Here's how the part is built. I have some questions about the finished solid (model axes, mm). Face numbers are marked on the shaded views. A direction names the side the tool comes from. Round coordinates to 2 decimals unless told otherwise and drop trailing zeros. Write each loop counter-clockwise with the first axis right and the second up, starting at its lowest first coordinate (ties: lowest second). Pieces come first, ordered by that corner, then holes. Notation, with made-up numbers: (27, 37) - (83, 37) arc R31 ccw to (83, 75) - close; hole circle Ø5 at (18, 17.25). An arc over 180 degrees is marked (long way). Write item = value, one per line. Start each with the question number.
Item 1: If we section it at D-D (x = 4): Please give me the cut outline in (y, z).
Item 2: If we section it at B-B (z = -88): Please give me the cut outline in (x, y), and give its area (3 significant figures).
Item 3: Which directions (+Z, -Z, +X, -X, +Y, -Y) give clear straight access to the entire face, cutting with the end or side of a thin tool? Please do the marked faces 1 and 2.
Item 4: If I drill on line 1 along X through (y, z) = (26, -39); line 2 along Y through (x, z) = (178, 8); line 3 along Z through (x, y) = (21, -136.5), over which ranges is the centre line in solid material (lowest first)? Write a range as [from, to].
Item 5: If we section it at A-A (x = -57.5): Please give me the cut outline in (y, z).
Item 6: For P1, Ø5, axis at x = -16, y = -50.5, coming from the -Z side; P2, Ø8, axis at y = -79.5, z = -106.5, coming from the -X side, each with a flat end and sliding along its axis, tell me the tip position at first contact or that it passes through.
Item 7: If we section it at C-C (y = -17.5): Please give me the cut outline in (x, z), and give its area (3 significant figures).
```python
from build123d import *

# Parameters (mm, degrees)
F0_W      = 406.4
F0_H      = 203.2
F1_DEPTH  = 101.6
F4_W      = 393.7
F4_H      = 190.5
F5_DEPTH  = 190.5
F6_R      = 38.1
F7_DEPTH  = 6.35
F10_DEPTH = 101.6


# Not quite as in the source:
# - the program builds the solid bodies; features that only make, move or delete a surface that nothing else refers to are left out


with BuildPart() as f1:
    # F0 (on Top) → F1 (new body, symmetric)
    with BuildSketch(Plane.XY):
        with Locations((-1.672681421, -62.5133958211)):
            Rectangle(F0_W, F0_H)
    extrude(amount=F1_DEPTH, both=True)

    # F4 (on offset) → F5 (cut)
    with BuildSketch(Plane.XZ.offset(157.7633958211)):
        with Locations((-1.672681421, 0)):
            Rectangle(F4_W, F4_H)
    extrude(amount=-F5_DEPTH, mode=Mode.SUBTRACT)

    # F6 (on face) → F7 (cut, through all)
    with BuildSketch(Plane(origin=(0, 0, -101.6), x_dir=(1, 0, 0), z_dir=(0, 0, -1))):
        with Locations((13.9572741464, 5.3633958211)):
            Circle(F6_R)
    extrude(amount=-F7_DEPTH, mode=Mode.SUBTRACT)

    # F9 (on offset) → F10 (join)
    with BuildSketch(Plane(origin=(0, 0, -95.25), x_dir=(1, 0, 0), z_dir=(0, 0, -1))):
        with BuildLine():
            ThreePointArc((13.9572742307, -32.7366041789), (40.8980425394, -21.5773725123), (52.0572741464, 5.3633958211))
            ThreePointArc((52.0572741464, 5.3633958211), (-12.9834942466, 32.3041641545), (13.9572742307, -32.7366041789))
        make_face()
    extrude(amount=F10_DEPTH)


solid = f1.part
```
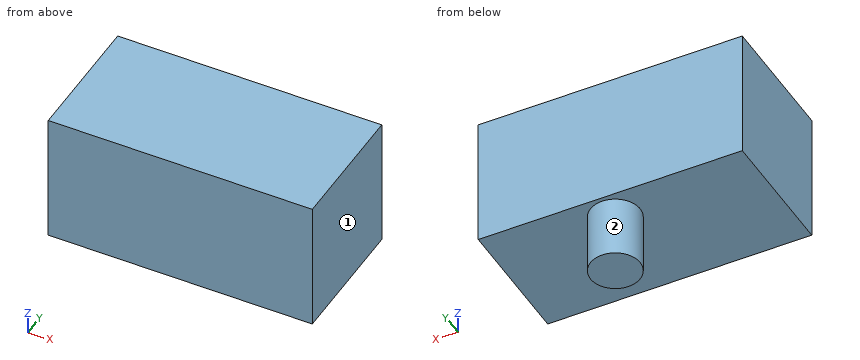
Reply:
q1.outline = (-164.11, -101.6) - (-42.14, -101.6) - (-42.14, -196.85) - (31.41, -196.85) - (31.41, -101.6) - (39.09, -101.6) - (39.09, 101.6) - (-164.11, 101.6) - close; hole (-157.76, -95.25) - (32.74, -95.25) - (32.74, 95.25) - (-157.76, 95.25) - close
q2.outline = (-204.87, -164.11) - (201.53, -164.11) - (201.53, 39.09) - (-204.87, 39.09) - close; hole (-198.52, -157.76) - (195.18, -157.76) - (195.18, 32.74) - (-198.52, 32.74) - close
q2.area = 7,580 mm2
q3.face_1 = +Z, -Z, +X, +Y, -Y
q3.face_2 = -Z
q4.line_1 = [-204.87, -198.52], [195.18, 201.53]
q4.line_2 = [-164.11, -157.76], [32.74, 39.09]
q4.line_3 = [-101.6, -95.25], [95.25, 101.6]
q5.outline = (-164.11, -101.6) - (39.09, -101.6) - (39.09, 101.6) - (-164.11, 101.6) - close; hole (-157.76, -95.25) - (32.74, -95.25) - (32.74, 95.25) - (-157.76, 95.25) - close
q6.P1 = -101.6
q6.P2 = through
q7.outline = (-204.87, -101.6) - (-22.16, -101.6) - (-22.16, -196.85) - (50.07, -196.85) - (50.07, -101.6) - (201.53, -101.6) - (201.53, 101.6) - (-204.87, 101.6) - close; hole (-198.52, -95.25) - (195.18, -95.25) - (195.18, 95.25) - (-198.52, 95.25) - close
q7.area = 14,500 mm2
